Can you work these out from the drawing? Everything is in mm from the part's minimum corner. A direction names the side the tool comes from. Coordinates: 2 decimals unless noted, no trailing zeros. Loops run counter-clockwise (first coordinate to the right, second up) from the corner with the lowest first, then second, coordinate; pieces in that order, holes last.
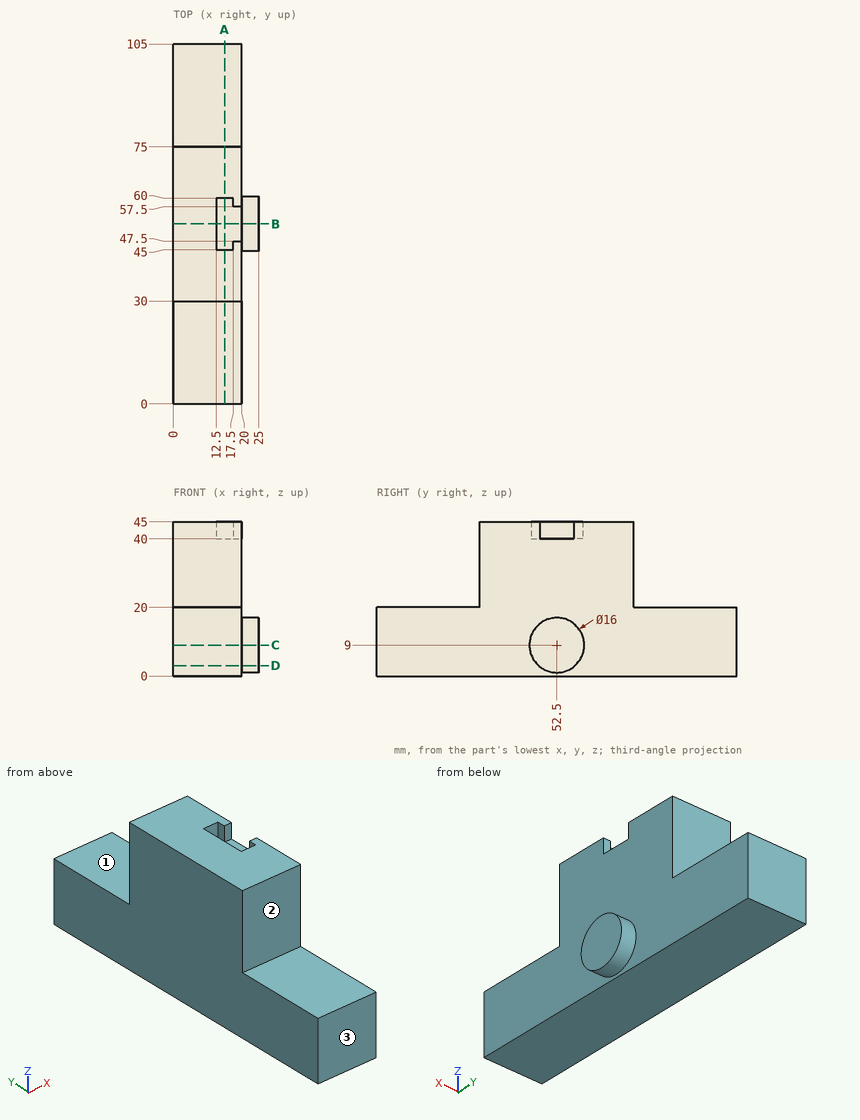
(1) Imagine slicing it at B-B, the plane y = 52.5. Write out the boundary of the cut face in (x, z).
Answers:
outline: (0, 0) - (20, 0) - (20, 1) - (25, 1) - (25, 17) - (20, 17) - (20, 40) - (12.5, 40) - (12.5, 45) - (0, 45) - close
(2) Which directions (+Z, -Z, +X, -X, +Y, -Y) give clear straight access to the entire face, cutting with the end or side of a thin tool? Please do the marked faces 1, 2 and 3.
Answers:
face 1: +Z, +X, -X, +Y
face 2: +Z, +X, -X, -Y
face 3: +Z, -Z, +X, -X, -Y
(3) Imagine slicing it at C-C, the plane z = 9. Write out the boundary of the cut face in (x, y), and give its area (3 significant figures).
Answers:
outline: (0, 0) - (20, 0) - (20, 44.5) - (25, 44.5) - (25, 60.5) - (20, 60.5) - (20, 105) - (0, 105) - close
area: 2,180 mm2
(4) Imagine slicing it at D-D, the plane z = 3. Write out the boundary of the cut face in (x, y), and give its area (3 significant figures).
Answers:
outline: (0, 0) - (20, 0) - (20, 47.21) - (25, 47.21) - (25, 57.79) - (20, 57.79) - (20, 105) - (0, 105) - close
area: 2,150 mm2
(5) I need wall thicknesses on probe 1 along Y at (x, z) = (8.5, 26.5); probe 2 along X at (y, z) = (71, 34). Which ranges of each line are inside material? Lowest first, please.
Answers:
probe 1: y = 30 to 75
probe 2: x = 0 to 20
(6) Imagine slicing it at A-A, the plane x = 15. Write out the boundary of the cut face in (y, z), and give its area (3 significant figures).
Answers:
outline: (0, 0) - (105, 0) - (105, 20) - (75, 20) - (75, 45) - (60, 45) - (60, 40) - (45, 40) - (45, 45) - (30, 45) - (30, 20) - (0, 20) - close
area: 3,150 mm2
(7) For pin 1 (8 mm diameter, centred on x = 11.5, z = 18, fed in from -Y); pin 2 (6 mm diameter, centred on x = 7, z = 27, fed in from -Y); pin 3 (10 mm diameter, centred on x = 7, z = 30.5, fed in from +Y); pin 4 (2.5 mm diameter, centred on y = 49, z = 42, fed in from +X), each with a flat end and sliding along its axis, tell me the tip position at first contact or that it passes through.
Answers:
pin 1: stops at y = 0
pin 2: stops at y = 30
pin 3: stops at y = 75
pin 4: stops at x = 12.5
